Read the model definition and answer for the solid it produces. Units are mm, in the model's axes. Face numbers are marked on the shaded views. A direction names the side the tool comes from. Coordinates: 2 decimals unless noted, no trailing zeros. Loops run counter-clockwise (first coordinate to the right, second up) from the corner with the lowest first, then second, coordinate; pieces in that order, holes last. Notation, with made-up numbers: M 33.25,52.5 L 61.25,52.5 A27 ccw 61.25,91.5 Z; hole C -15.75,-3.75 d8. An arc over 180 degrees is marked long. Use one line per item in the form item = value. Start each with the question number.
1. Flat-ended cylindrical pins translate along their axes: pin 1 (3 mm diameter, centred on x = 5, z = 1.5, fed in from +Y); pin 2 (3 mm diameter, centred on x = -6, y = 5, fed in from -Z). Find the tip coordinate at first contact, or state that the pin passes through.
2. Find the intervals of material crossed by probe 1 along X at (y, z) = (1.1, 5); probe 2 along X at (y, z) = (2.5, 11.25); probe 3 along Y at (x, z) = (10.75, 7.75), in increasing order. Write a range as [from, to].
3. The part is cut by section A-A (z = 4). Give the vertices of the cut face in (x, y).
4. The part is cut by section C-C (y = 1). Give the vertices of the cut face in (x, z).
5. For a pull along Z with two mould halves and no side action, classify the marked faces 1, 2 and 3 as released by +Z, released by -Z, zero draft, split by the parting line, or undercut.
6. A tool of negligible diameter and unlimited length cuts with its end or side. For the marked faces 4, 5 and 6, from which of +Z, -Z, +X, -X, +Y, -Y can it reach the whole face along a straight path? Write none if from no direction.
7. The part is cut by section B-B (x = 2.25). Give the vertices of the cut face in (y, z), plus the area to 3 significant figures.
8. The part is cut by section D-D (x = -5.5). Give the vertices of the cut face in (y, z).
from build123d import *

# Parameters (mm, degrees)
T_LE_DE_BASE_PLI_E1_DEPTH = 12
ENL_V_START               = 7
ENL_V_MAT_EXTRU_1_DEPTH   = 5
ESQUISSE7_R               = 1.75
ENL_V_MAT_EXTRU_2_DEPTH   = 10
CONG_1_R                  = 5.2


# Read off the part's stored shape, not the designer's step: Enlèv. mat.-Extru.1
# Sheet-metal steps are written as plain solids
with BuildPart() as part:
    # Esquisse1 → Tôle de base pliée1 (new body)
    with BuildSketch(Plane(origin=(0, 0, 0), x_dir=(0, 0, -1), z_dir=(1, 0, 0))):
        with BuildLine():
            Line((0, 0), (-10.354560188, 0))
            ThreePointArc((-10.354560188, 0), (-12.295688846, 1.243807141), (-11.976787844, 3.527080849))
            Line((-11.976787844, 3.527080849), (-9, 7))
            Line((-9, 7), (-7.937040757, 6.088892077))
            Line((-7.937040757, 6.088892077), (-10.913828601, 2.615972926))
            ThreePointArc((-10.913828601, 2.615972926), (-11.023770789, 1.828806674), (-10.354560188, 1.4))
            Line((-10.354560188, 1.4), (0, 1.4))
            Line((0, 1.4), (0, 0))
        make_face()
    extrude(amount=T_LE_DE_BASE_PLI_E1_DEPTH)

    # Enlèv. mat.-Extru.1 outline → Enlèv. mat.-Extru.1 (cut)
    with BuildSketch(Plane.YZ.offset(ENL_V_START)):
        with BuildLine():
            Line((0, 10.354560188), (1.4, 10.354560188))
            ThreePointArc((1.4, 10.354560188), (1.828806674, 11.023770789), (2.615972926, 10.913828601))
            Line((2.615972926, 10.913828601), (6.088892077, 7.937040757))
            Line((6.088892077, 7.937040757), (7, 9))
            Line((7, 9), (3.527080849, 11.976787844))
            ThreePointArc((3.527080849, 11.976787844), (1.243807141, 12.295688846), (0, 10.354560188))
        make_face()
    extrude(amount=ENL_V_MAT_EXTRU_1_DEPTH, mode=Mode.SUBTRACT)

    # Esquisse7 → Enlèv. mat.-Extru.2 (cut)
    with BuildSketch(Plane(origin=(0, 1.4, 0), x_dir=(1, 0, 0), z_dir=(0, 1, 0))):
        with Locations(Location((7, -5, 0), (0, 0, 270))):
            Circle(ESQUISSE7_R)
    extrude(amount=-ENL_V_MAT_EXTRU_2_DEPTH, mode=Mode.SUBTRACT)

    # Congé1
    # the kernel refuses this fillet: 5.2 mm, written as the material it takes off along each edge
    with BuildSketch(Plane(origin=(12, -12.990381057, 10.354560188), x_dir=(-1, 0, 0), z_dir=(0, 1, 0))) as cong_1_piece_1:
        with BuildLine():
            CenterArc((5.2, -5.196152423), CONG_1_R, 92.204227504, 87.795772496)
            Line((0, -5.196152423), (-0.104, -5.196152423))
            Line((-0.104, -5.196152423), (-0.104, 0))
            Line((-0.104, 0), (0, 0.104))
            ThreePointArc((0, 0.104), (2.5, 0.104), (4.996, 0.103923048))
            Line((4.996, 0.103923048), (5, 0))
        make_face()
    extrude(amount=27.380762114, mode=Mode.SUBTRACT)
    with BuildSketch(Plane(origin=(12, 14.4, 0), x_dir=(-1, 0, 0), z_dir=(0, -1, 0))) as cong_1_piece_2:
        with BuildLine():
            CenterArc((CONG_1_R, -CONG_1_R), CONG_1_R, 90, 90)
            Line((0, -CONG_1_R), (-CONG_1_R * 0.02, -CONG_1_R))
            Line((-CONG_1_R * 0.02, -CONG_1_R), (-CONG_1_R * 0.02, CONG_1_R * 0.02))
            Line((-CONG_1_R * 0.02, CONG_1_R * 0.02), (CONG_1_R, CONG_1_R * 0.02))
            Line((CONG_1_R, CONG_1_R * 0.02), (CONG_1_R, 0))
        make_face()
    extrude(amount=27.4, mode=Mode.SUBTRACT)

    # Symétrie1: part across plane


with BuildPart() as part_1:
    add(part.part)
    add(part.part.mirror(Plane(origin=(0, 2.615972926, 10.913828601), x_dir=(0, 0, 1), z_dir=(-1, 0, 0))))


solid = part_1.part
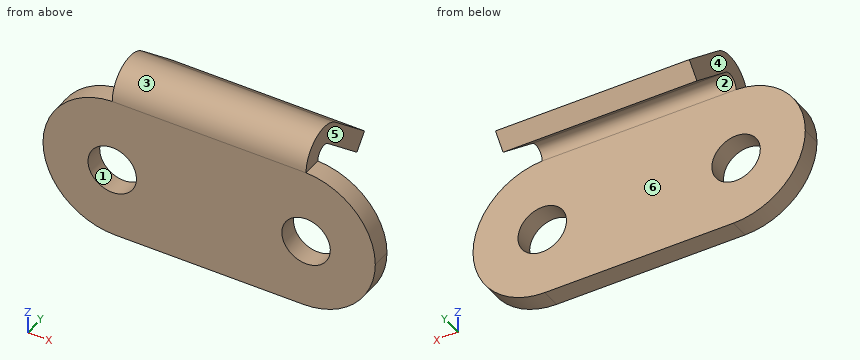
Computed values:
q1.pin_1 = 1.4
q1.pin_2 = 7.94
q2.probe_1 = [-12, -8.75], [-5.25, 5.25], [8.75, 12]
q2.probe_2 = [-7, 7]
q2.probe_3 = [0, 1.4]
q3.outline = M -11.86,0 L -8.44,0 L -8.44,1.4 L -11.86,1.4 Z; M -5.56,0 L 5.56,0 L 5.56,1.4 L -5.56,1.4 Z; M 8.44,0 L 11.86,0 L 11.86,1.4 L 8.44,1.4 Z
q4.outline = M -12,5.18 A5.2 ccw -6.8,0 L 6.8,0 A5.2 ccw 12,5.18 A5.2 ccw 7,10.35 L 7,12.16 L -7,12.16 L -7,10.35 A5.2 ccw Z; hole C -7,5 d3.5; hole C 7,5 d3.5
q5.face_1 = undercut
q5.face_2 = released by -Z
q5.face_3 = released by +Z
q6.face_4 = +Z, -X, +Y
q6.face_5 = +Z, +X, +Y
q6.face_6 = -Z, +X, -X
q7.outline = M 0,0 L 1.4,0 L 1.4,10.35 A0.74 cw 2.62,10.91 L 6.09,7.94 L 7,9 L 3.53,11.98 A2.14 ccw 0,10.35 Z
q7.area = 25.5 mm²
q8.outline = M 0,0 L 1.4,0 L 1.4,4.1 L 0,4.1 Z; M 0,5.9 L 1.4,5.9 L 1.4,10.35 A0.74 cw 2.62,10.91 L 6.09,7.94 L 7,9 L 3.53,11.98 A2.14 ccw 0,10.35 Z
